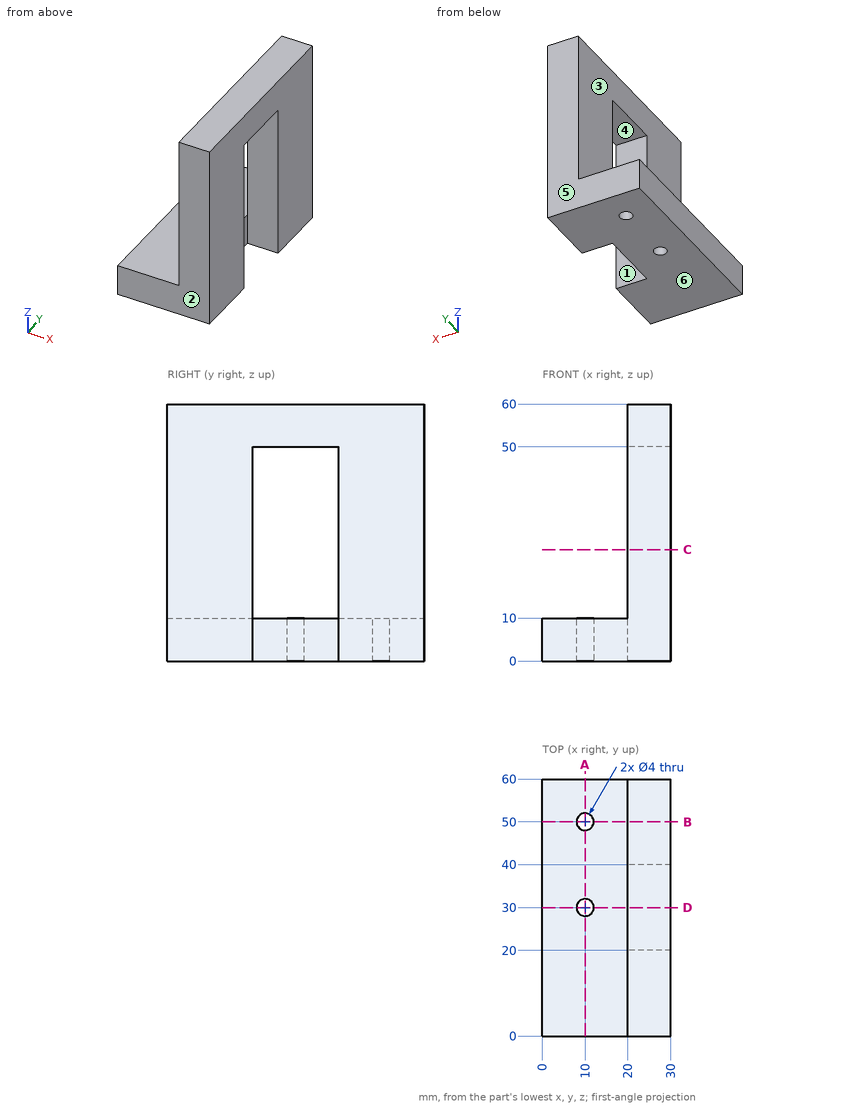
Check sheet for the drawn part. Datum: minimum x, y, z corner. Units: mm. A direction names the side the tool comes from. Coordinates: 2 decimals unless noted, no trailing zeros. Order: outer loops, then holes, each group sorted by start corner. A loop starts at its lowest first (then second) coordinate and runs counter-clockwise, first axis right, second up. Notation, with made-up numbers: M 40.25,12 L 89.25,12 A13 cw 89.25,33 Z; hole C 36,17 d4. An arc over 180 degrees is marked long. One line per item, written item: value. Start each with the question number.
Item 1: Mould release check, pull along Y, two halves, no side actions. Record for the marked faces 4, 5 and 6: released by +Y, released by -Y, zero draft, split by the parting line, or undercut.
Item 2: Sectioned sample at A-A (x = 10). Enter the section's corners in (y, z).
Item 3: Access from +Z, -Z, +X, -X, +Y, -Y to the whole of each face (thin tool, end or side, straight path). Record for the marked faces 1, 2 and 3.
Item 4: Sectioned sample at D-D (y = 30). Enter the section's corners in (x, z).
Item 5: Sectioned sample at C-C (z = 26). Enter the section's corners in (x, y), then the cut area to 3 significant figures.
Item 6: Scan lines: probe 1 along Y at (x, z) = (10, 4); probe 2 along Y at (x, z) = (22.5, 40.5); probe 3 along Z at (x, y) = (23.75, 27.5). Record each from-to range of solid material in increasing order.
Item 7: Gauge pin test, flat ends, axial feed: pin 1 (1 mm diameter, centred on x = 16, y = 15.5, fed in from +Z); pin 2 (5 mm diameter, centred on x = 26, y = 32, fed in from -Z); pin 3 (8 mm diameter, centred on y = 31, z = 5.5, fed in from +X). Record the tip position at first contact, or that the pin passes through.
Item 8: Sectioned sample at B-B (y = 50). Enter the section's corners in (x, z), then the cut area to 3 significant figures.
Conclusion:
1. face 4: undercut
1. face 5: released by +Y
1. face 6: zero draft
2. outline: M 0,0 L 28,0 L 28,10 L 0,10 Z; M 32,0 L 48,0 L 48,10 L 32,10 Z; M 52,0 L 60,0 L 60,10 L 52,10 Z
3. face 1: -Z, +X
3. face 2: +Z, -Z, +X, -X, -Y
3. face 3: +Z, -X, +Y, -Y
4. outline: M 0,0 L 8,0 L 8,10 L 0,10 Z; M 12,0 L 20,0 L 20,10 L 12,10 Z; M 20,50 L 30,50 L 30,60 L 20,60 Z
5. outline: M 20,0 L 30,0 L 30,20 L 20,20 Z; M 20,40 L 30,40 L 30,60 L 20,60 Z
5. area: 400 mm^2
6. probe 1: y = 0 to 28, 32 to 48, 52 to 60
6. probe 2: y = 0 to 20, 40 to 60
6. probe 3: z = 50 to 60
7. pin 1: stops at z = 10
7. pin 2: stops at z = 50
7. pin 3: stops at x = 20
8. outline: M 0,0 L 8,0 L 8,10 L 0,10 Z; M 12,0 L 30,0 L 30,60 L 20,60 L 20,10 L 12,10 Z
8. area: 760 mm^2
